```python
from build123d import *

# Parameters (mm, degrees)
SKETCH_1_W          = 18
SKETCH_1_H          = 10
EXTRUDE_1_DEPTH     = 70
SKETCH_2_R          = 2
CUT_EXTRUDE_1_DEPTH = 11
SKETCH_3_R          = 2
CUT_EXTRUDE_2_DEPTH = 19


with BuildPart() as part:
    # 草图1 → 凸台-拉伸1 (new body)
    with BuildSketch(Plane.XY):
        Rectangle(SKETCH_1_W, SKETCH_1_H)
    extrude(amount=EXTRUDE_1_DEPTH)

    # 草图2 → 切除-拉伸1 (cut, through all)
    with BuildSketch(Plane(origin=(0, 5, 0), x_dir=(1, 0, 0), z_dir=(0, 1, 0))):
        with Locations((0, -5)):
            Circle(SKETCH_2_R)
        with Locations((0, -35)):
            Circle(SKETCH_2_R)
        with Locations((0, -65)):
            Circle(SKETCH_2_R)
    extrude(amount=-CUT_EXTRUDE_1_DEPTH, mode=Mode.SUBTRACT)

    # 草图3 → 切除-拉伸2 (cut, through all)
    with BuildSketch(Plane(origin=(9, 0, 0), x_dir=(0, 0, -1), z_dir=(1, 0, 0))):
        with Locations((-50, 0)):
            Circle(SKETCH_3_R)
        with Locations((-20, 0)):
            Circle(SKETCH_3_R)
    extrude(amount=-CUT_EXTRUDE_2_DEPTH, mode=Mode.SUBTRACT)


solid = part.part
```
Geometry: final body of the model. Coordinates: model frame, mm. Round coordinates to 2 decimals unless told otherwise and drop trailing zeros. Order: outer loops, then holes, each group sorted by start corner. A loop starts at its lowest first (then second) coordinate and runs counter-clockwise, first axis right, second up. Notation, with made-up numbers: (-23.75, 41.5) - (-10.75, 41.5) arc R19 ccw to (-10.75, 57.5) - close; hole circle Ø7 at (49, 81.5). An arc over 180 degrees is marked (long way). Use CSV: the item, a comma, the result in double quotes. Start each with the question number.
Q1. Mould query, pull axis Z, two halves, no side actions, for faces 1 (the face through (-9, 0, 35)), 2 (the face through (0, 0, 63)), 3 (the face through (0, 0, 0)). Classes: +Z half, -Z half, draft (parallel to the pull), parting line (faces both ways), or undercut.
Q2. Material intervals for line 1 along X through (y, z) = (-1.5, 5); line 2 along Z through (x, y) = (0, -2.75); line 3 along Z through (x, y) = (4.75, -1.5), sorted ascending. Write a range as from..to.
Q3. Section query D-D (y = 2.75). Return loops of the section in (x, z).
Q4. Section query B-B (z = 20). Return loops of the section in (x, y), and give its area (3 significant figures).
Q5. Section query A-A (y = 0). Return loops of the section in (x, z), and give its area (3 significant figures).
Q6. First-contact query: pin 1 (2.5 mm diameter, centred on y = 0, z = 50, fed in from -X). Flat tip, straight axial feed; report the tip coordinate or a pass-through.
Q7. Section query C-C (x = -4.25). Return loops of the section in (y, z).
Result set:
1,face 1,"draft"
1,face 2,"undercut"
1,face 3,"-Z half"
2,line 1,"x = -9..-2, 2..9"
2,line 2,"z = 0..3, 7..33, 37..63, 67..70"
2,line 3,"z = 0..18.68, 21.32..48.68, 51.32..70"
3,outline,"(-9, 0) - (9, 0) - (9, 70) - (-9, 70) - close; hole circle Ø4 at (0, 5); hole circle Ø4 at (0, 35); hole circle Ø4 at (0, 65)"
4,outline,"(-9, -5) - (9, -5) - (9, -2) - (-9, -2) - close; (-9, 2) - (9, 2) - (9, 5) - (-9, 5) - close"
4,area,"108 mm2"
5,outline,"(-9, 0) - (9, 0) - (9, 18) - (-9, 18) - close; (-9, 22) - (9, 22) - (9, 48) - (-9, 48) - close; (-9, 52) - (9, 52) - (9, 70) - (-9, 70) - close; hole circle Ø4 at (0, 5); hole circle Ø4 at (0, 35); hole circle Ø4 at (0, 65)"
5,area,"1,080 mm2"
6,pin 1,"passes through"
7,outline,"(-5, 0) - (5, 0) - (5, 70) - (-5, 70) - close; hole circle Ø4 at (0, 20); hole circle Ø4 at (0, 50)"
